from build123d import *

# Parameters (mm, degrees)
SKETCH1_R               = 2.5
BOSS_EXTRUDE1_DEPTH     = 6
CUT_EXTRUDE1_DEPTH      = 60.673537378
CUT_EXTRUDE1_DEPTH_BACK = 3
SKETCH2_R               = 2.5


with BuildPart() as part:
    # Sketch1 → Boss-Extrude1 (new body)
    # profile 1 of 2: a face of its own
    with BuildSketch(Plane.XY):
        with BuildLine():
            ThreePointArc((30, -5), (35, 0), (30, 5))
            Line((30, 5), (0, 5))
            ThreePointArc((0, 5), (-5, 0), (0, -5))
            Line((0, -5), (30, -5))
        make_face()
        with Locations((30, 0)):
            Circle(SKETCH1_R, mode=Mode.SUBTRACT)
        Circle(SKETCH1_R, mode=Mode.SUBTRACT)
    # profile 2 of 2: a face of its own
    with BuildSketch(Plane.XY):
        with BuildLine():
            Line((35, -42.957596512), (35, 0))
            ThreePointArc((35, 0), (33.535533906, -3.535533906), (30, -5))
            Line((30, -5), (11.394465816, -5))
            Line((11.394465816, -5), (11.394465816, -23.685159648))
            Line((11.394465816, -23.685159648), (25.817798964, -45.697887462))
            ThreePointArc((25.817798964, -45.697887462), (31.429859227, -47.748786613), (35, -42.957596512))
        make_face()
    extrude(amount=BOSS_EXTRUDE1_DEPTH)

    # Sketch2 → Cut-Extrude1 (cut, two sides: drawn at the far end of the back side and taken through both)
    with BuildSketch(Plane.XY.offset(6).offset(-CUT_EXTRUDE1_DEPTH_BACK)):
        with BuildLine():
            Line((30, 5), (15.828754387, 5))
            Line((15.828754387, 5), (15.828754387, -8.999149352))
            Line((15.828754387, -8.999149352), (35, -8.999149352))
            Line((35, -8.999149352), (35, 0))
            ThreePointArc((35, 0), (33.535533906, 3.535533906), (30, 5))
        make_face()
        with Locations((30, 0)):
            Circle(SKETCH2_R, mode=Mode.SUBTRACT)
    extrude(amount=CUT_EXTRUDE1_DEPTH + CUT_EXTRUDE1_DEPTH_BACK, mode=Mode.SUBTRACT)


solid = part.part
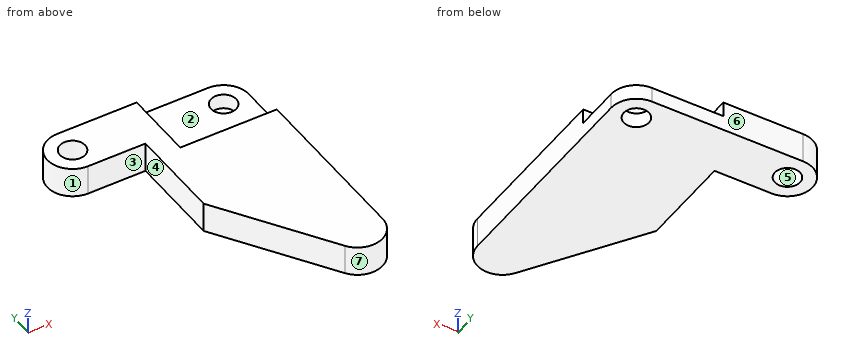
Input: part model. Units: mm. Frame: model coordinates. Face numbers are marked on the shaded views. A direction names the side the tool comes from. Coordinates: 2 decimals unless noted, no trailing zeros. Loops run counter-clockwise (first coordinate to the right, second up) from the corner with the lowest first, then second, coordinate; pieces in that order, holes last.
Q1. Cut plane B-B (x = 3.5). Output: boundary loops of the cut face in (y, z).
Q2. Cut plane C-C (y = -23). Output: boundary loops of the cut face in (x, z), then the cut area to 3 significant figures.
Q3. Cut plane A-A (z = 2.35). Output: boundary loops of the cut face in (x, y), then the cut area to 3 significant figures.
Q4. Material intervals for line 1 (Y direction, x = 0, z = 2.2); line 2 (Y direction, x = 30, z = 0.65); line 3 (X direction, y = 1, z = 4.7), sorted ascending.
Q5. Contact query for flat-ended pins moving along their axis: pin 1 (3 mm diameter, centred on y = -35, z = 4, fed in from -X); pin 2 (1.8 mm diameter, centred on x = 6, z = 4, fed in from -Y); pin 3 (8 mm diameter, centred on x = 30, y = 0, fed in from +Z). Output: stop coordinate, or through.
Q6. Draft query along Y for the marked faces 4, 5, 6 and 7. Return one class per face: +Y half, -Y half, draft (parallel to the pull), parting line (faces both ways), or undercut.
Q7. Set-up query: the marked faces 1, 2 and 3. Return all of +Z, -Z, +X, -X, +Y, -Y with unobstructed straight access to the full face (end or side cutting, diameter ignored); none if empty.
Working result:
1. outline: (-5, 0) - (5, 0) - (5, 6) - (-5, 6) - close
2. outline: (11.39, 0) - (35, 0) - (35, 6) - (11.39, 6) - close
2. area: 142 mm2
3. outline: (0, -5) - (11.39, -5) - (11.39, -23.69) - (25.82, -45.7) arc R5 ccw to (35, -42.96) - (35, 0) arc R5 ccw to (30, 5) - (0, 5) arc R5 ccw to start; hole circle Ø5 at (0, 0); hole circle Ø5 at (30, 0)
3. area: 1,160 mm2
4. line 1: y = -5 to -2.5, 2.5 to 5
4. line 2: y = -47.96 to -2.5, 2.5 to 5
4. line 3: x = -4.9 to -2.29, 2.29 to 15.83
5. pin 1: stops at x = 17.83
5. pin 2: stops at y = -5
5. pin 3: stops at z = 3
6. face 4: draft
6. face 5: undercut
6. face 6: +Y half
6. face 7: -Y half
7. face 1: +Z, -Z, -X
7. face 2: +Z, +X, +Y
7. face 3: +Z, -Z, -X, -Y
